Check sheet for the modelled part. Datum: model origin and axes. Units: mm. A direction names the side the tool comes from. Round coordinates to 2 decimals unless told otherwise and drop trailing zeros. Write each loop counter-clockwise with the first axis right and the second up, starting at its lowest first coordinate (ties: lowest second). Pieces come first, ordered by that corner, then holes. Notation, with made-up numbers: (0.5, -33.75) -> (33.5, -33.75) arc R32 cw to (33.5, -5.75) -> close; hole circle Ø6 at (43, 84.25). An arc over 180 degrees is marked (long way). Put each result on its own line as item: value. Start each with the question number.
from build123d import *

# Parameters (mm, degrees)
SKETCH2_R           = 30
BOSS_EXTRUDE1_DEPTH = 150
SKETCH3_R           = 20
CUT_EXTRUDE1_DEPTH  = 100
SKETCH4_W           = 25
SKETCH4_H           = 20
BOSS_EXTRUDE2_DEPTH = 50
SKETCH5_R           = 7.5
CUT_EXTRUDE2_DEPTH  = 40


with BuildPart() as part:
    # Sketch2 → Boss-Extrude1 (new body)
    with BuildSketch(Plane(origin=(0, 0, 0), x_dir=(1, 0, 0), z_dir=(0, 1, 0))):
        with Locations(Location((0, 0, 0), (0, 0, 270))):
            Circle(SKETCH2_R)
    extrude(amount=BOSS_EXTRUDE1_DEPTH)

    # Sketch3 → Cut-Extrude1 (cut)
    with BuildSketch(Plane(origin=(0, 0, 0), x_dir=(0, 0, -1), z_dir=(1, 0, 0))):
        with Locations((0, 50)):
            Circle(SKETCH3_R)
    extrude(amount=-CUT_EXTRUDE1_DEPTH, mode=Mode.SUBTRACT)

    # Sketch4 → Boss-Extrude2 (add)
    with BuildSketch(Plane(origin=(0, 150, 0), x_dir=(1, 0, 0), z_dir=(0, 1, 0))):
        Rectangle(SKETCH4_W, SKETCH4_H)
    extrude(amount=BOSS_EXTRUDE2_DEPTH)

    # Sketch5 → Cut-Extrude2 (cut)
    with BuildSketch(Plane(origin=(0, 0, -10), x_dir=(-1, 0, 0), z_dir=(0, 0, -1))):
        with Locations((0, 180)):
            Circle(SKETCH5_R)
    extrude(amount=-CUT_EXTRUDE2_DEPTH, mode=Mode.SUBTRACT)


solid = part.part
1. Material ranges on L1, parallel to Y at x = -11, z = -0.5; L2, parallel to Y at x = -15, z = 0; L3, parallel to Y at x = 4, z = -18, recorded low to high. Write a range as [from, to].
2. Access from +Z, -Z, +X, -X, +Y, -Y to the whole of each face (thin tool, end or side, straight path). Record for faces 4 (the flat face through (-12.5, 175, 0)), 5 (the flat face through (12.5, 175, 0)), 6 (the flat face through (0, 50, 0)), 7 (the flat face through (0, 169, 10)).
3. Section check C-C, the plane z = 0. Enter the section's corners in (x, y).
4. Gauge pin test, flat ends, axial feed: P1, Ø19.5, axis at x = 0, y = 180, coming from the -Z side; P2, Ø6, axis at x = 20.5, y = 100.5, coming from the +Z side; P3, Ø1.5, axis at x = -8, y = 155, coming from the +Z side; P4, Ø10, axis at x = -16, z = 7.5, coming from the +Y side. Record the tip position at first contact, or that the pin passes through.
5. Draft check along Y on faces 1 (the flat face through (0, 200, 0)), 2 (the cylindrical face through (-15, 38, 16)), 3 (the flat face through (0, 169, -10)). Enter one of: released by +Y, released by -Y, zero draft, split by the parting line, or undercut.
6. Section check B-B, the plane x = 2. Enter the section's corners in (y, z).
7. Section check A-A, the plane y = 180. Enter the section's corners in (x, z).
8. Section check D-D, the plane x = -15. Enter the section's corners in (y, z).
Reply:
1. L1: y = [0, 30.01], [69.99, 200]
1. L2: y = [0, 30], [70, 150]
1. L3: y = [0, 150]
2. face 4: +Z, -Z, -X, +Y
2. face 5: +Z, -Z, +X, +Y
2. face 6: -X
2. face 7: +Z, +X, -X, +Y
3. outline: (-30, 0) -> (30, 0) -> (30, 150) -> (12.5, 150) -> (12.5, 200) -> (-12.5, 200) -> (-12.5, 150) -> (-30, 150) -> (-30, 70) -> (0, 70) -> (0, 30) -> (-30, 30) -> close; hole circle Ø15 at (0, 180)
4. P1: stops at z = -10
4. P2: stops at z = 24.37
4. P3: stops at z = 10
4. P4: stops at y = 200
5. face 1: released by +Y
5. face 2: undercut
5. face 3: zero draft
6. outline: (0, -29.93) -> (150, -29.93) -> (150, -10) -> (172.77, -10) -> (172.77, 10) -> (150, 10) -> (150, 29.93) -> (0, 29.93) -> close; (187.23, -10) -> (200, -10) -> (200, 10) -> (187.23, 10) -> close
7. outline: (-12.5, -10) -> (-7.5, -10) -> (-7.5, 10) -> (-12.5, 10) -> close; (7.5, -10) -> (12.5, -10) -> (12.5, 10) -> (7.5, 10) -> close
8. outline: (0, -25.98) -> (150, -25.98) -> (150, 25.98) -> (0, 25.98) -> close; hole circle Ø40 at (50, 0)
